```python
from build123d import *

# Parameters (mm, degrees)
F1_DEPTH = 25
F3_DEPTH = 20
F4_R     = 2.5
F5_DEPTH = 25.001


with BuildPart() as f1:
    # F0 (on Right) → F1 (new body)
    with BuildSketch(Plane.YZ):
        with BuildLine():
            Line((-22.5, -35), (22.5, -35))
            ThreePointArc((22.5, -35), (36.792858, 0), (22.5, 35))
            Line((22.5, 35), (-22.5, 35))
            ThreePointArc((-22.5, 35), (-36.792858, 0), (-22.5, -35))
        make_face()
    extrude(amount=F1_DEPTH)

    # F2 (on face) → F3 (cut)
    with BuildSketch(Plane.YZ.offset(25)):
        Polygon((28.145826, -16.25), (28.145826, 16.25), (0, 32.5), (-28.145826, 16.25), (-28.145826, -16.25), (0, -32.5), align=None)
    extrude(amount=-F3_DEPTH, mode=Mode.SUBTRACT)

    # F4 (on face) → F5 (cut, through all)
    with BuildSketch(Plane.YZ.offset(25)):
        with Locations((-20, 30)):
            Circle(F4_R)
        with Locations((20, 30)):
            Circle(F4_R)
        with Locations((20, -30)):
            Circle(F4_R)
        with Locations((-20, -30)):
            Circle(F4_R)
    extrude(amount=-F5_DEPTH, mode=Mode.SUBTRACT)


solid = f1.part
```
Geometry: final body of the model. Coordinates: model frame, mm. A direction names the side the tool comes from. Round coordinates to 2 decimals unless told otherwise and drop trailing zeros. Write each loop counter-clockwise with the first axis right and the second up, starting at its lowest first coordinate (ties: lowest second). Pieces come first, ordered by that corner, then holes. Notation, with made-up numbers: (86.25, -35) -> (105.25, -35) arc R28 cw to (105.25, -5) -> close; hole circle Ø1 at (87, -16.5). An arc over 180 degrees is marked (long way). Use CSV: the item, a comma, the result in double quotes. Start each with the question number.
Q1. Section A-A (x = 21.75). Return loops of the section in (y, z), plus the area to 3 significant figures.
Q2. Section B-B (y = 20). Return loops of the section in (x, z).
Q3. Reachability of faces 4 (the face through (12, 0, 35)), 5 (the face through (15.14, -14.27, -24.26)) from +Z, -Z, +X, -X, +Y, -Y: full face, straight path, thin tool, end or side. Return the list, or none.
Q4. First-contact query: pin 1 Ø2 at (x, z) = (22, -1.5) entering from +Y; pin 2 Ø5 at (y, z) = (25.5, -14.5) entering from -X; pin 3 Ø8 at (x, y) = (11, -29.5) entering from -Z; pin 4 Ø3 at (y, z) = (1, 3.5) entering from +X. Flat tips, straight axial feed; report the tip coordinate or a pass-through.
Q5. Section C-C (z = -30). Return loops of the section in (x, y).
Q6. Line query: L1, parallel to Z at x = 19.5, y = -20; L2, parallel to Z at x = 9.75, y = 1.5; L3, parallel to Y at x = 8, z = -18. Output: solid intervals per line, ascending.
Q7. Section D-D (y = -24). Return loops of the section in (x, z), plus the area to 3 significant figures.
Q8. Pull-direction query (Z, two-part tool) for faces 1 (the face through (12.32, 36.79, -0.54)), 2 (the face through (12.68, 18.16, -28.31)), 3 (the face through (12, 0, -35)); classes: pulls with the +Z half, pulls with the -Z half, needs draft (parallel to the pull), parting line crosses it, or undercut.
Result sheet:
1,outline,"(-22.5, -35) -> (22.5, -35) arc R50 ccw to (22.5, 35) -> (-22.5, 35) arc R50 ccw to start; hole (-28.15, -16.25) -> (0, -32.5) -> (28.15, -16.25) -> (28.15, 16.25) -> (0, 32.5) -> (-28.15, 16.25) -> close; hole circle Ø5 at (-20, -30); hole circle Ø5 at (-20, 30); hole circle Ø5 at (20, -30); hole circle Ø5 at (20, 30)"
1,area,"1,700 mm²"
2,outline,"(0, -35) -> (25, -35) -> (25, -32.5) -> (0, -32.5) -> close; (0, -27.5) -> (25, -27.5) -> (25, -20.95) -> (5, -20.95) -> (5, 20.95) -> (25, 20.95) -> (25, 27.5) -> (0, 27.5) -> close; (0, 32.5) -> (25, 32.5) -> (25, 35) -> (0, 35) -> close"
3,face 4,"+Z, +X, -X, +Y, -Y"
3,face 5,"+X"
4,pin 1,"y = 36.79"
4,pin 2,"x = 0"
4,pin 3,"z = -31.65"
4,pin 4,"x = 5"
5,outline,"(0, -26.79) -> (25, -26.79) -> (25, -22.5) -> (0, -22.5) -> close; (0, -17.5) -> (25, -17.5) -> (25, -4.33) -> (5, -4.33) -> (5, 4.33) -> (25, 4.33) -> (25, 17.5) -> (0, 17.5) -> close; (0, 22.5) -> (25, 22.5) -> (25, 26.79) -> (0, 26.79) -> close"
6,L1,"-35 to -32.5, -27.5 to -20.95, 20.95 to 27.5, 32.5 to 35"
6,L2,"-35 to -31.63, 31.63 to 35"
6,L3,"-33.44 to -25.11, 25.11 to 33.44"
7,outline,"(0, -33.4) -> (25, -33.4) -> (25, -18.64) -> (5, -18.64) -> (5, 18.64) -> (25, 18.64) -> (25, 33.4) -> (0, 33.4) -> close"
7,area,"924 mm²"
8,face 1,"parting line crosses it"
8,face 2,"undercut"
8,face 3,"pulls with the -Z half"
